Geometry check sheet. Reference: drawing and pictorial views, mm from the part's lowest x, y, z. A direction names the side the tool comes from. Coordinates: 2 decimals unless noted, no trailing zeros. Loops run counter-clockwise (first coordinate to the right, second up) from the corner with the lowest first, then second, coordinate; pieces in that order, holes last. Notation, with made-up numbers: (-5.75, 21) -> (37.25, 21) arc R18 cw to (37.25, 46) -> close; hole circle Ø10 at (32, 41.25). An arc over 180 degrees is marked (long way). Answer as a JSON object with one key per item and string values. Group by question number.
Q1. Gauge pin test, flat ends, axial feed: pin 1 Ø8 at (y, z) = (27.5, 53.5) entering from +X; pin 2 Ø0.6 at (y, z) = (4.5, 19) entering from -X; pin 3 Ø1.5 at (x, y) = (18.5, 28) entering from -Z. Record the tip position at first contact, or that the pin passes through.
Q2. Release check for a two-part mould opening along Y. For the marked faces 3, 4 and 5 record: released by +Y, released by -Y, zero draft, split by the parting line, or undercut.
Q3. Set-up check for the marked faces 1 and 2: record each of +Z, -Z, +X, -X, +Y, -Y from which the full face is reachable in a straight line by a thin tool's end or side.
Q4. Cross-section at C-C on z = 30. Record the boundary of the cut face in (x, y).
Q5. Cross-section at A-A on x = 54. Record the boundary of the cut face in (y, z).
Q6. Scan lines: L1, parallel to Y at x = 19.5, z = 37.5; L2, parallel to Y at x = 4, z = 17.5; L3, parallel to Z at x = 17, y = 13.5. Record each from-to range of solid material in increasing order.
Q7. Cross-section at D-D on x = 30. Record the boundary of the cut face in (y, z), and give its area (3 significant figures).
Q8. Cross-section at B-B on z = 54. Record the boundary of the cut face in (x, y), and give its area (3 significant figures).
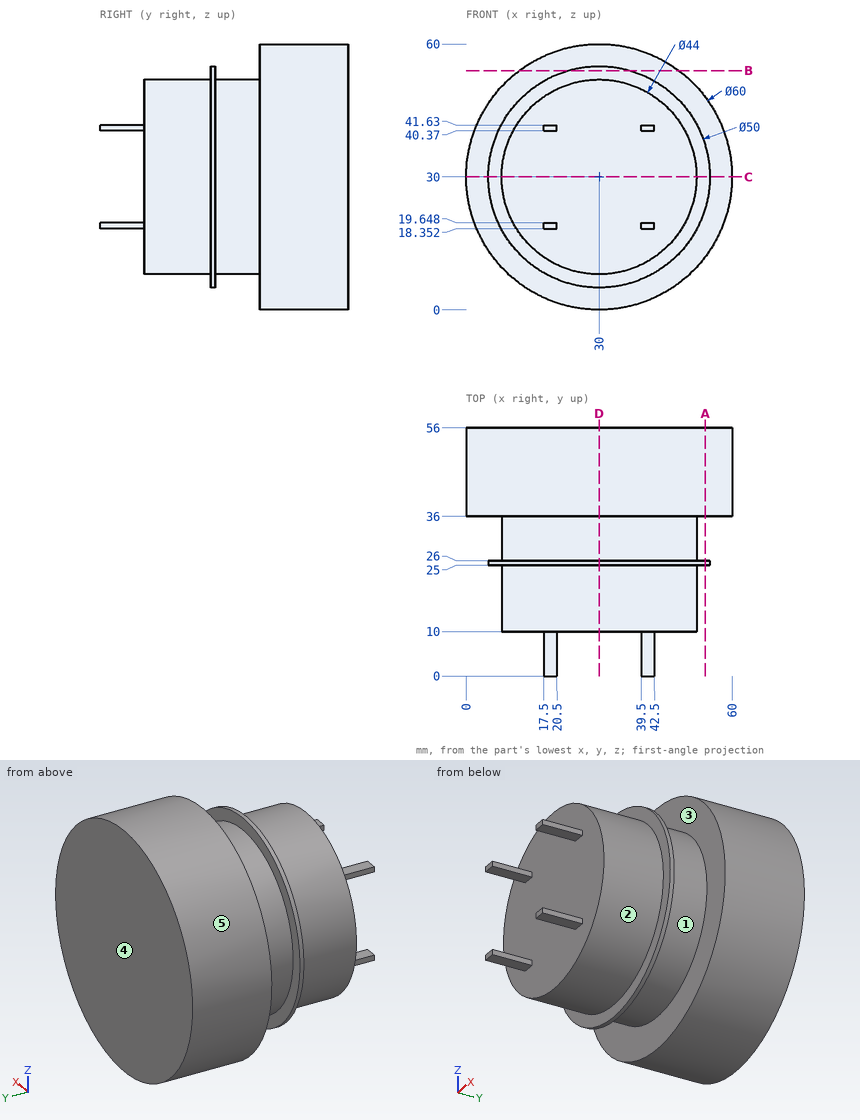
Computed values:
{
 "1": {"pin 1": "stops at x = 45.27", "pin 2": "stops at x = 17.5", "pin 3": "stops at z = 10.81"},
 "2": {"face 3": "undercut", "face 4": "released by +Y", "face 5": "zero draft"},
 "3": {"face 1": "none", "face 2": "-Y"},
 "4": {"outline": "(0, 36) -> (8, 36) -> (8, 26) -> (5, 26) -> (5, 25) -> (8, 25) -> (8, 10) -> (52, 10) -> (52, 25) -> (55, 25) -> (55, 26) -> (52, 26) -> (52, 36) -> (60, 36) -> (60, 56) -> (0, 56) -> close"},
 "5": {"outline": "(25, 23) -> (26, 23) -> (26, 37) -> (25, 37) -> close; (36, 12) -> (56, 12) -> (56, 48) -> (36, 48) -> close"},
 "6": {"L1": "y = 10 to 56", "L2": "y = 36 to 56", "L3": "z = 12.25 to 47.75"},
 "7": {"outline": "(10, 8) -> (25, 8) -> (25, 5) -> (26, 5) -> (26, 8) -> (36, 8) -> (36, 0) -> (56, 0) -> (56, 60) -> (36, 60) -> (36, 52) -> (26, 52) -> (26, 55) -> (25, 55) -> (25, 52) -> (10, 52) -> close", "area": "2,350 mm²"},
 "8": {"outline": "(12, 36) -> (48, 36) -> (48, 56) -> (12, 56) -> close; (23, 25) -> (37, 25) -> (37, 26) -> (23, 26) -> close", "area": "734 mm²"}
}
